Autodesk Inventor part; units mm, degrees
ref_plane "YZ Plane" through (0, 0, 0) normal (1, 0, 0) x (0, 1, 0)
ref_plane "XZ Plane" through (0, 0, 0) normal (0, 1, 0) x (-1, 0, 0)
ref_plane "XY Plane" through (0, 0, 0) normal (0, 0, 1) x (1, 0, 0)
ref_plane "Arbeitsebene1" through (0, 0, 0) normal (0, 0, 1) x (1, 0, 0)
sketch "Skizze1" plane through (0, 0, 0) normal (0, 0, 1) x (1, 0, 0)
  arc A0 (9.5966, 13.5152) -> (9.0972, 14.0928) centre (8.4862, 13.06) ccw construction
  arc A1 (8.9755, 14.2862) -> (9.0972, 14.0928) centre (9.2245, 14.308) ccw construction
  line L0 (8.9755, 14.2862) -> (8.9453, 14.6318) construction
  arc A2 (8.9453, 14.6318) -> (8.6962, 14.86) centre (8.6962, 14.61) ccw construction
  line L1 (8.6962, 14.86) -> (8.2438, 14.86) construction
  arc A3 (8.2438, 14.86) -> (7.9947, 14.6318) centre (8.2438, 14.61) ccw construction
  line L2 (7.9947, 14.6318) -> (7.9627, 14.2652) construction
  arc A4 (7.8468, 14.0755) -> (7.9627, 14.2652) centre (7.7136, 14.287) ccw construction
  arc A5 (7.8468, 14.0755) -> (7.3759, 13.5152) centre (8.4862, 13.06) ccw construction
  arc A6 (7.1446, 13.36) -> (7.3759, 13.5152) centre (7.1446, 13.61) ccw construction
  line L3 (7.1446, 13.36) -> (6.47, 13.36) construction
  line L4 (6.47, 13.36) -> (5.97, 13.86) construction
  line L5 (5.97, 13.86) -> (5.97, 24.86) construction
  line L6 (5.97, 24.86) -> (6.47, 25.36) construction
  line L7 (6.47, 25.36) -> (7.1446, 25.36) construction
  arc A7 (7.3759, 25.2048) -> (7.1446, 25.36) centre (7.1446, 25.11) ccw construction
  arc A8 (7.3759, 25.2048) -> (7.8468, 24.6445) centre (8.4862, 25.66) ccw construction
  arc A9 (7.9627, 24.4548) -> (7.8468, 24.6445) centre (7.7136, 24.433) ccw construction
  line L8 (7.9627, 24.4548) -> (7.9947, 24.0882) construction
  arc A10 (7.9947, 24.0882) -> (8.2438, 23.86) centre (8.2438, 24.11) ccw construction
  line L9 (8.2438, 23.86) -> (8.6962, 23.86) construction
  arc A11 (8.6962, 23.86) -> (8.9453, 24.0882) centre (8.6962, 24.11) ccw construction
  line L10 (8.9453, 24.0882) -> (8.9755, 24.4338) construction
  arc A12 (9.0972, 24.6272) -> (8.9755, 24.4338) centre (9.2245, 24.412) ccw construction
  arc A13 (9.0972, 24.6272) -> (9.5966, 25.2048) centre (8.4862, 25.66) ccw construction
  arc A14 (9.8279, 25.36) -> (9.5966, 25.2048) centre (9.8279, 25.11) ccw construction
  line L11 (9.8279, 25.36) -> (10.97, 25.36) construction
  line L12 (10.97, 25.36) -> (10.97, 32.26) construction
  line L13 (10.97, 32.26) -> (10.37, 32.86) construction
  line L14 (10.37, 32.86) -> (6.97, 32.86) construction
  arc A15 (6.17, 32.86) -> (6.97, 32.86) centre (6.57, 33.16) ccw construction
  line L15 (6.17, 32.86) -> (1.57, 32.86) construction
  line L16 (1.57, 32.86) -> (0.97, 32.26) construction
  line L17 (0.97, 32.26) -> (0.97, 25.76) construction
  line L18 (0.97, 25.76) -> (1.37, 25.36) construction
  line L19 (1.37, 25.36) -> (1.37, 13.36) construction
  line L20 (1.37, 13.36) -> (0.97, 12.96) construction
  line L21 (0.97, 12.96) -> (0.97, 6.46) construction
  line L22 (0.97, 6.46) -> (1.57, 5.86) construction
  line L23 (1.57, 5.86) -> (10.37, 5.86) construction
  line L24 (10.37, 5.86) -> (10.97, 6.46) construction
  line L25 (10.97, 6.46) -> (10.97, 13.36) construction
  line L26 (10.97, 13.36) -> (9.8279, 13.36) construction
  arc A16 (9.5966, 13.5152) -> (9.8279, 13.36) centre (9.8279, 13.61) ccw construction
  line L27 (10.4528, 5.66) -> (1.4872, 5.66) construction
  line L28 (1.4872, 5.66) -> (0.77, 6.3772) construction
  line L29 (0.77, 6.3772) -> (0.77, 13.0428) construction
  line L30 (0.77, 13.0428) -> (1.17, 13.4428) construction
  line L31 (1.17, 13.4428) -> (1.17, 25.2772) construction
  line L32 (1.17, 25.2772) -> (0.77, 25.6772) construction
  line L33 (0.77, 25.6772) -> (0.77, 32.3428) construction
  line L34 (0.77, 32.3428) -> (1.4872, 33.06) construction
  line L35 (1.4872, 33.06) -> (6.2872, 33.06) construction
  arc A17 (6.2872, 33.06) -> (6.8528, 33.06) centre (6.57, 33.16) ccw construction
  line L36 (6.8528, 33.06) -> (10.4528, 33.06) construction
  line L37 (10.4528, 33.06) -> (11.17, 32.3428) construction
  line L38 (11.17, 32.3428) -> (11.17, 25.16) construction
  line L39 (11.17, 25.16) -> (9.8279, 25.16) construction
  arc A18 (9.8279, 25.16) -> (9.7816, 25.129) centre (9.8279, 25.11) ccw construction
  arc A19 (9.1991, 24.4551) -> (9.7816, 25.129) centre (8.4862, 25.66) ccw construction
  arc A20 (9.1991, 24.4551) -> (9.1747, 24.4164) centre (9.2245, 24.412) ccw construction
  line L40 (9.1747, 24.4164) -> (9.1445, 24.0708) construction
  arc A21 (8.6962, 23.66) -> (9.1445, 24.0708) centre (8.6962, 24.11) ccw construction
  line L41 (8.6962, 23.66) -> (8.2438, 23.66) construction
  arc A22 (7.7955, 24.0708) -> (8.2438, 23.66) centre (8.2438, 24.11) ccw construction
  line L42 (7.7955, 24.0708) -> (7.7634, 24.4373) construction
  arc A23 (7.7634, 24.4373) -> (7.7403, 24.4753) centre (7.7136, 24.433) ccw construction
  arc A24 (7.1909, 25.129) -> (7.7403, 24.4753) centre (8.4862, 25.66) ccw construction
  arc A25 (7.1909, 25.129) -> (7.1446, 25.16) centre (7.1446, 25.11) ccw construction
  line L43 (7.1446, 25.16) -> (6.5528, 25.16) construction
  line L44 (6.5528, 25.16) -> (6.17, 24.7772) construction
  line L45 (6.17, 24.7772) -> (6.17, 13.9428) construction
  line L46 (6.17, 13.9428) -> (6.5528, 13.56) construction
  line L47 (6.5528, 13.56) -> (7.1446, 13.56) construction
  arc A26 (7.1446, 13.56) -> (7.1909, 13.591) centre (7.1446, 13.61) ccw construction
  arc A27 (7.7403, 14.2447) -> (7.1909, 13.591) centre (8.4862, 13.06) ccw construction
  arc A28 (7.7403, 14.2447) -> (7.7634, 14.2827) centre (7.7136, 14.287) ccw construction
  line L48 (7.7634, 14.2827) -> (7.7955, 14.6492) construction
  arc A29 (8.2438, 15.06) -> (7.7955, 14.6492) centre (8.2438, 14.61) ccw construction
  line L49 (8.2438, 15.06) -> (8.6962, 15.06) construction
  arc A30 (9.1445, 14.6492) -> (8.6962, 15.06) centre (8.6962, 14.61) ccw construction
  line L50 (9.1445, 14.6492) -> (9.1747, 14.3036) construction
  arc A31 (9.1747, 14.3036) -> (9.1991, 14.2649) centre (9.2245, 14.308) ccw construction
  arc A32 (9.7816, 13.591) -> (9.1991, 14.2649) centre (8.4862, 13.06) ccw construction
  arc A33 (9.7816, 13.591) -> (9.8279, 13.56) centre (9.8279, 13.61) ccw construction
  line L51 (9.8279, 13.56) -> (11.17, 13.56) construction
  line L52 (11.17, 13.56) -> (11.17, 6.3772) construction
  line L53 (11.17, 6.3772) -> (10.4528, 5.66) construction
  line L54 (11.17, 25.66) -> (33.0091, 25.66)
  line L55 (11.17, 25.66) -> (33.0091, 25.66) construction
  line L56 (33.0091, 33.86) -> (15.3197, 33.86)
  line L57 (15.3197, 33.86) -> (11.1197, 38.06)
  line L58 (11.1197, 38.06) -> (0.1946, 38.06)
  line L59 (-16.23, 33.06) -> (-16.23, 19.36)
  line L60 (-16.23, 19.36) -> (1.17, 19.36)
  line L61 (1.17, 19.36) -> (1.17, 25.2772)
  line L62 (1.17, 25.2772) -> (0.77, 25.6772)
  line L63 (0.77, 25.6772) -> (0.77, 33.06)
  line L64 (0.77, 33.06) -> (11.17, 33.06)
  line L65 (11.17, 33.06) -> (11.17, 25.66)
  line L66 (36.7731, 34.36) -> (36.7731, 25.3561)
  line L67 (36.7731, 13.415) -> (36.7731, 4.36)
  line L68 (0.1946, 38.06) -> (-4.8054, 33.06)
  line L69 (0.1946, 38.06) -> (7.2656, 38.06) construction
  line L70 (-4.8054, 33.06) -> (-16.23, 33.06)
  line L71 (33.0091, 33.86) -> (33.0091, 25.66)
  line L72 (33.0091, 33.86) -> (61.0424, 33.86)
  line L73 (61.0424, 33.86) -> (61.0424, 19.36)
  line L74 (61.0424, 19.36) -> (57.0424, 19.36)
  line L75 (37.0424, 19.36) -> (27.0424, 19.36)
  line L76 (27.0424, 19.36) -> (27.0424, 25.66)
  circle A34 centre (47.0424, 19.36) radius 10
  point P0 (0, 0)
  point P1 (-2.0031, 19.36)
  point P2 (-4.8031, 19.36)
  dimension "d0" = 0.2
  dimension "d2" = 5
  dimension "d4" = 17
  dimension "d7" = 0.5
  dimension "d8" = 3.5
  dimension "d21" = 135
  dimension "d45" = 20
  dimension "d46" = 14
  dimension "d47" = 20
  dimension "d48" = 14.5
extrude "Extrusion1" add sketch "Skizze1" along normal blind 8 contours L65 L64 L63 L62 L61 L60 L59 L70 L68 L58 L57 L56 L71 L54 | L54 L71 L72 L73 L74 A34 L75 L76
sketch "Skizze2" plane through (-16.23, 19.36, 0) normal (-1, 0, 0) x (0, 0, 1)
  circle A0 centre (5, 10) radius 1.75
  line L0 (0, 13.7) -> (0, 0)
  line L1 (0, 0) -> (8, 0)
  line L2 (8, 13.7) -> (8, 0)
  line L3 (0, 13.7) -> (8, 13.7)
  circle A1 centre (5, 10) radius 1.5
  point P0 (0, -19.36)
  dimension "d11" = 3
hole "Bohrung1" at (-16.23, 29.36, 5) direction (1, 0, 0) diameter 3 depth 20 tip angle 118 counterbore diameter 6 counterbore depth 4
mirror "Spiegeln2" about plane through (-16.23, 19.36, 0) normal (0, -1, 0) of "Extrusion1", "Bohrung1"
sketch "Skizze6" plane through (0, 0, 8) normal (0, 0, 1) x (1, 0, 0)
  line L0 (-16.23, 33.06) -> (-16.23, 5.66)
  circle A0 centre (-8.2208, 19.4223) radius 1.9812
  circle A1 centre (-8.2208, 19.4223) radius 8.0094
  point P0 (0, 0)
  point P1 (-16.23, 19.36)
extrude "Extrusion5" add sketch "Skizze6" along normal blind 14 contours A0 | A1
sketch "Skizze7" plane through (0, 0, 0) normal (0, 0, -1) x (-1, 0, 0)
  circle A0 centre (8.2208, 19.4223) radius 6
  circle A1 centre (8.2208, 19.4223) radius 1.9812
  point P0 (0, 0)
  dimension "d34" = 12
extrude "Extrusion6" cut sketch "Skizze7" against normal blind 20 contours A0 | A1
sketch "Skizze8" plane through (-7.7141, 19.36, 22) normal (0, 0, 1) x (1, 0, 0)
  circle A0 centre (-0.5067, 0.0623) radius 1.5
  circle A1 centre (-0.5067, 0.0623) radius 1.4224
  point P0 (7.7141, -19.36)
  dimension "d37" = 3
extrude "Extrusion7" cut sketch "Skizze8" against normal blind 15 contours A0 | A1
fillet "Rundung1" radius 5 9 edges at (61.0424, 33.86, 4) (61.0424, 4.86, 4) (11.1197, 0.66, 4) (0.1946, 0.66, 4) (-4.8054, 5.66, 4) (15.3197, 33.86, 4) (11.1197, 38.06, 4) (0.1946, 38.06, 4) (-4.8054, 33.06, 4)
properties part number "30_Cube_Cube_Z_Focus_NEMA8_captive_objectivemount_v0"
Work out the finished part from the listing and answer in its coordinate system (mm). A direction names the side the tool comes from. Round coordinates to 2 decimals unless told otherwise and drop trailing zeros. Write each loop counter-clockwise with the first axis right and the second up, starting at its lowest first coordinate (ties: lowest second). Pieces come first, ordered by that corner, then holes. Notation, with made-up numbers: (-33, 21) - (-4, 21) arc R18 cw to (-4, 35) - close; hole circle Ø2 at (-16, 24). An arc over 180 degrees is marked (long way). Answer in a Markdown table with one row per item. Add a question column.
1. A cutting plane is placed at A-A, the plane y = 24.5. Determine the outline of the cut face in (x, z), and give its area (3 significant figures).
2. Given pin 1 (6.5 mm diameter, centred on x = -10.5, z = 4.5, fed in from -Y); pin 2 (1.5 mm diameter, centred on x = 40.5, z = 4, fed in from -Y); pin 3 (3.5 mm diameter, centred on y = 9.36, z = 5, fed in from -X); pin 4 (2.5 mm diameter, centred on x = -8.22, y = 19.42, fed in from -Z), each flat-ended and moving along its own axis, determine where each tip first touches the part or whether it passes through.
3. A cutting plane is placed at C-C, the plane z = 2.75. Count the separate pieces of the cut face and the enclosed holes in it, and give its area (3 significant figures).
4. A cutting plane is placed at B-B, the plane x = 7.5. Determine the outline of the cut face in (y, z), and give its area (3 significant figures).
5. For faces 1 (the cylindrical face through (-5.64, 10.69, 5.69)), 2 (the flat face through (0.77, 29, 3)), 3 (the flat face through (-12, 5.66, 4)), determine the directions among +Z, -Z, +X, -X, +Y, -Y from which every point of the face is accessible in a straight line to the end or side of a thin tool.
6. A cutting plane is placed at D-D, the plane x = 35.5. Determine the outline of the cut face in (y, z).
7. The mould has two halves that part along X. Classify faces 4 (the flat face through (6, 0.66, 4)), 5 (the flat face through (6, 5.66, 4)), 6 (the cylindrical face through (15.45, 34.25, 4.06)): +X half, -X half, draft (parallel to the pull), parting line (faces both ways), or undercut.
8. Find the intervals of material crossed by line 1 along Y through (x, z) = (-14.4, 5); line 2 along Y through (x, z) = (4.5, 3.25); line 3 along Y through (x, z) = (-8.75, 5), in increasing order. Write a range as from..to.
Worked out:
| question | item | result |
|---|---|---|
| 1 | outline | (-16.23, 0) - (-11.42, 0) - (-11.42, 20) - (-5.02, 20) - (-5.02, 0) - (1.17, 0) - (1.17, 8) - (-2.03, 8) - (-2.03, 22) - (-14.41, 22) - (-14.41, 8) - (-16.23, 8) - close; (27.04, 0) - (38.46, 0) - (38.46, 8) - (27.04, 8) - close; (55.62, 0) - (61.04, 0) - (61.04, 8) - (55.62, 8) - close |
| 1 | area | 320 mm^2 |
| 2 | pin 1 | y = 5.66 |
| 2 | pin 2 | y = 4.86 |
| 2 | pin 3 | x = -12.23 |
| 2 | pin 4 | through |
| 3 | separate pieces | 1 |
| 3 | enclosed holes | 3 |
| 3 | area | 1,400 mm^2 |
| 4 | outline | (0.66, 0) - (5.66, 0) - (5.66, 8) - (0.66, 8) - close; (33.06, 0) - (38.06, 0) - (38.06, 8) - (33.06, 8) - close |
| 4 | area | 80.0 mm^2 |
| 5 | face 1 | -X |
| 5 | face 2 | +Z, -Z |
| 5 | face 3 | +Z, -Z, -X, -Y |
| 6 | outline | (4.86, 0) - (33.86, 0) - (33.86, 8) - (4.86, 8) - close |
| 7 | face 4 | draft |
| 7 | face 5 | undercut |
| 7 | face 6 | +X half |
| 8 | line 1 | 5.66..6.36, 12.36..26.36, 32.36..33.06 |
| 8 | line 2 | 0.66..5.66, 33.06..38.06 |
| 8 | line 3 | 5.66..7.86, 10.86..13.45, 25.4..27.86, 30.86..33.06 |
